from build123d import *

# Parameters (mm, degrees)
F1_DEPTH  = 14
F3_DEPTH  = 7
F4_R      = 10
F5_R      = 5
F6_R      = 2.6
F7_DEPTH  = 14.001
F8_R      = 5
F9_DEPTH  = 5
F10_W     = 26
F10_H     = 6
F11_DEPTH = 13
F12_W     = 40
F12_H     = 4
F13_DEPTH = 6


with BuildPart() as f1:
    # F0 (on Top) → F1 (new body)
    with BuildSketch(Plane.XY):
        Polygon((137.5, -71.5), (167.5, -71.5), (167.5, 71.5), (-167.5, 71.5), (-167.5, -71.5), (-137.5, -71.5), (-137.5, -96.5), (137.5, -96.5), align=None)
        with BuildLine():
            ThreePointArc((147.5, -49), (146.767767, -50.767767), (145, -51.5))
            Line((145, -51.5), (-145, -51.5))
            ThreePointArc((-145, -51.5), (-146.767767, -50.767767), (-147.5, -49))
            Line((-147.5, -49), (-147.5, 49))
            ThreePointArc((-147.5, 49), (-146.767767, 50.767767), (-145, 51.5))
            Line((-145, 51.5), (145, 51.5))
            ThreePointArc((145, 51.5), (146.767767, 50.767767), (147.5, 49))
            Line((147.5, 49), (147.5, -49))
        make_face(mode=Mode.SUBTRACT)
    extrude(amount=F1_DEPTH)

    # F2 (on face) → F3 (cut)
    with BuildSketch(Plane(origin=(0, 0, 0), x_dir=(1, 0, 0), z_dir=(0, 0, -1))):
        with BuildLine():
            Line((-145, -57.5), (145, -57.5))
            ThreePointArc((145, -57.5), (151.010408, -55.010408), (153.5, -49))
            Line((153.5, -49), (153.5, 49))
            ThreePointArc((153.5, 49), (151.010408, 55.010408), (145, 57.5))
            Line((145, 57.5), (-145, 57.5))
            ThreePointArc((-145, 57.5), (-151.010408, 55.010408), (-153.5, 49))
            Line((-153.5, 49), (-153.5, -49))
            ThreePointArc((-153.5, -49), (-151.010408, -55.010408), (-145, -57.5))
        make_face()
        with BuildLine():
            Line((147.5, 49), (147.5, -49))
            ThreePointArc((147.5, -49), (146.767767, -50.767767), (145, -51.5))
            Line((145, -51.5), (-145, -51.5))
            ThreePointArc((-145, -51.5), (-146.767767, -50.767767), (-147.5, -49))
            Line((-147.5, -49), (-147.5, 49))
            ThreePointArc((-147.5, 49), (-146.767767, 50.767767), (-145, 51.5))
            Line((-145, 51.5), (145, 51.5))
            ThreePointArc((145, 51.5), (146.767767, 50.767767), (147.5, 49))
        make_face(mode=Mode.SUBTRACT)
    extrude(amount=-F3_DEPTH, mode=Mode.SUBTRACT)

    # F4
    f4_edges = [f1.edges().sort_by_distance(p)[0] for p in [
        (-167.5, -71.5, 7),
        (167.5, -71.5, 7),
        (137.5, -96.5, 7),
        (-137.5, -96.5, 7),
        (167.5, 71.5, 7),
        (-167.5, 71.5, 7),
    ]]
    fillet(f4_edges, radius=F4_R)

    # F5
    f5_edges = [f1.edges().sort_by_distance(p)[0] for p in [
        (137.5, -71.5, 7),
        (-137.5, -71.5, 7),
    ]]
    fillet(f5_edges, radius=F5_R)

    # F6 (on face) → F7 (cut, through all)
    with BuildSketch(Plane.XY.offset(14)):
        with Locations((0, -81.5)):
            Circle(F6_R)
        with Locations((-100, -81.5)):
            Circle(F6_R)
        with Locations((100, -81.5)):
            Circle(F6_R)
    extrude(amount=-F7_DEPTH, mode=Mode.SUBTRACT)

    # F8 (on face) → F9 (cut)
    with BuildSketch(Plane.XY.offset(14)):
        with Locations((-100, -81.5)):
            Circle(F8_R)
        with Locations((0, -81.5)):
            Circle(F8_R)
        with Locations((100, -81.5)):
            Circle(F8_R)
    extrude(amount=-F9_DEPTH, mode=Mode.SUBTRACT)

    # F10 (on face) → F11 (join)
    with BuildSketch(Plane(origin=(0, 71.5, 0), x_dir=(-1, 0, 0), z_dir=(0, 1, 0))):
        with Locations((-102.5, 11)):
            Rectangle(F10_W, F10_H)
        with Locations((-7.5, 11)):
            Rectangle(F10_W, F10_H)
        with Locations((87.5, 11)):
            Rectangle(F10_W, F10_H)
    extrude(amount=F11_DEPTH)

    # F12 (on face) → F13 (join)
    with BuildSketch(Plane.XY.offset(14)):
        with Locations((-87.5, 73.5)):
            Rectangle(F12_W, F12_H)
        with Locations((7.5, 73.5)):
            Rectangle(F12_W, F12_H)
        with Locations((102.5, 73.5)):
            Rectangle(F12_W, F12_H)
    extrude(amount=-F13_DEPTH)


solid = f1.part
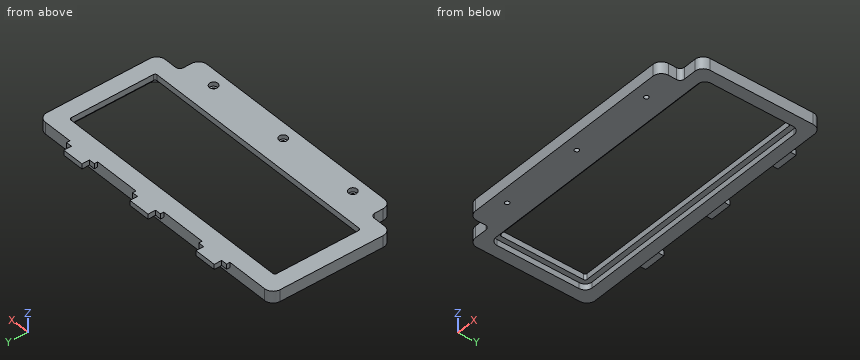
Geometry: final body of the model. Coordinates: model frame, mm. Give positions to 0.01 mm unless a question says otherwise; leave off trailing zeros. Write each loop counter-clockwise with the first axis right and the second up, starting at its lowest first coordinate (ties: lowest second). Pieces come first, ordered by that corner, then holes. Notation, with made-up numbers: M -24,51 L 19,51 A8 cw 19,63 Z; hole C -34,13.5 d1. An arc over 180 degrees is marked long. Answer in a Markdown table with one row per item. Add a question column.
(1) Section A-A on y = -7.5. Return loops of the section in (x, z).
(2) Section B-B on x = -41. Return loops of the section in (y, z).
(3) First-contact query: pin 1 (5 mm diameter, centred on y = 81.5, z = 12, fed in from +X); pin 2 (4 mm diameter, centred on x = 100, y = -81.5, fed in from +Z); pin 3 (1 mm diameter, centred on x = 60, y = -77.5, fed in from -Z); pin 4 (5 mm diameter, centred on x = -125.5, z = 12.5, fed in from +Y). Flat tips, straight axial feed; report the tip coordinate or a pass-through.
(4) Ray query, line 1 (Y direction, x = 0, z = 12.35); line 2 (X direction, y = -18, z = 10.5); line 3 (Y direction, x = -103, z = 5). Return the intervals inside material, ascending.
(5) Section C-C on z = 2.25. Return loops of the section in (x, y), and give its area (3 significant figures).
Result set:
| question | item | result |
|---|---|---|
| 1 | outline | M -167.5,0 L -153.5,0 L -153.5,7 L -147.5,7 L -147.5,14 L -167.5,14 Z; M 147.5,7 L 153.5,7 L 153.5,0 L 167.5,0 L 167.5,14 L 147.5,14 Z |
| 2 | outline | M -96.5,0 L -57.5,0 L -57.5,7 L -51.5,7 L -51.5,14 L -96.5,14 Z; M 51.5,7 L 57.5,7 L 57.5,0 L 71.5,0 L 71.5,14 L 51.5,14 Z |
| 3 | pin 1 | stops at x = 115.5 |
| 3 | pin 2 | passes through |
| 3 | pin 3 | stops at z = 0 |
| 3 | pin 4 | stops at y = 71.5 |
| 4 | line 1 | y = -96.5 to -86.5, -76.5 to -51.5, 51.5 to 84.5 |
| 4 | line 2 | x = -167.5 to -147.5, 147.5 to 167.5 |
| 4 | line 3 | y = -96.5 to -57.5, 57.5 to 71.5 |
| 5 | outline | M -167.5,-61.5 A10 ccw -157.5,-71.5 L -142.5,-71.5 A5 cw -137.5,-76.5 L -137.5,-86.5 A10 ccw -127.5,-96.5 L 127.5,-96.5 A10 ccw 137.5,-86.5 L 137.5,-76.5 A5 cw 142.5,-71.5 L 157.5,-71.5 A10 ccw 167.5,-61.5 L 167.5,61.5 A10 ccw 157.5,71.5 L -157.5,71.5 A10 ccw -167.5,61.5 Z; hole M -153.5,-49 A8.5 ccw -145,-57.5 L 145,-57.5 A8.5 ccw 153.5,-49 L 153.5,49 A8.5 ccw 145,57.5 L -145,57.5 A8.5 ccw -153.5,49 Z; hole C -100,-81.5 d5.2; hole C 0,-81.5 d5.2; hole C 100,-81.5 d5.2 |
| 5 | area | 19,400 mm^2 |
